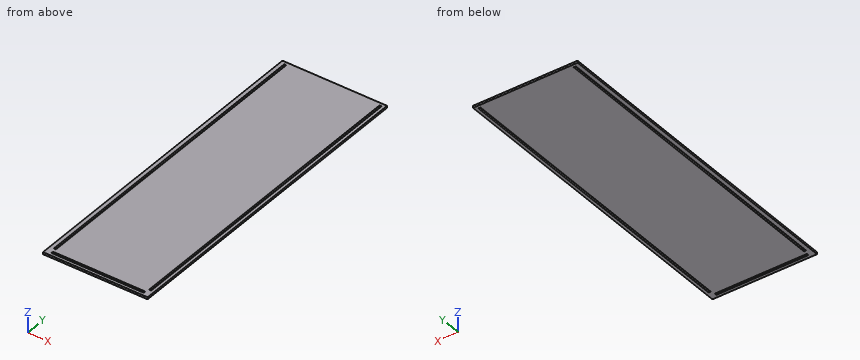
from build123d import *

# Parameters (mm, degrees)
F0_W     = 8.73125
F0_H     = 1295.4
F1_DEPTH = 8.73125


with BuildPart() as f1:
    # F0 (on Top) → F1 (new body)
    with BuildSketch(Plane.XY):
        Polygon((215.9, 673.1), (-215.9, 673.1), (-215.9, -673.1), (0, -673.1), (215.9, -673.1), (215.9, 74.258551), align=None)
        Polygon((190.5, -660.4), (0, -660.4), (-190.5, -660.4), (-190.5, -651.66875), (190.5, -651.66875), align=None, mode=Mode.SUBTRACT)
        with Locations((-194.865625, 12.70608)):
            Rectangle(F0_W, F0_H, mode=Mode.SUBTRACT)
        Polygon((203.2, 660.4), (203.2, 74.258551), (203.2, -635), (194.46875, -634.99392), (194.46875, 660.4), align=None, mode=Mode.SUBTRACT)
    extrude(amount=F1_DEPTH)


solid = f1.part
Can you work these out from the model? Positions are in its coordinate system, mm. Round coordinates to 2 decimals unless told otherwise and drop trailing zeros. Order: outer loops, then holes, each group sorted by start corner. A loop starts at its lowest first (then second) coordinate and runs counter-clockwise, first axis right, second up. Notation, with made-up numbers: (82.25, -25.5) -> (94.25, -25.5) arc R19 ccw to (94.25, -5.5) -> close; hole circle Ø4 at (16, 74.25). An arc over 180 degrees is marked (long way). Write each question's results on one line, items separated by ' | '. Start each with the question number.
Item 1: Please list where these lines run through material, in increasing order: L1, parallel to X at y = -428, z = 6; L2, parallel to Y at x = -162, z = 5.25; L3, parallel to Y at x = -192, z = 0.75.
Item 2: If we section it at A-A, the plane z = 6.75: Write out the boundary of the cut face in (x, y).
Item 3: If we section it at B-B, the plane y = -448: Write out the boundary of the cut face in (x, z).
Results:
1) L1: x = -215.9 to -199.23, -190.5 to 194.47, 203.2 to 215.9 | L2: y = -673.1 to -660.4, -651.67 to 673.1 | L3: y = -673.1 to -634.99, 660.41 to 673.1
2) outline: (-215.9, -673.1) -> (215.9, -673.1) -> (215.9, 673.1) -> (-215.9, 673.1) -> close; hole (-199.23, -634.99) -> (-190.5, -634.99) -> (-190.5, 660.41) -> (-199.23, 660.41) -> close; hole (-190.5, -660.4) -> (190.5, -660.4) -> (190.5, -651.67) -> (-190.5, -651.67) -> close; hole (194.47, -634.99) -> (203.2, -635) -> (203.2, 660.4) -> (194.47, 660.4) -> close
3) outline: (-215.9, 0) -> (-199.23, 0) -> (-199.23, 8.73) -> (-215.9, 8.73) -> close; (-190.5, 0) -> (194.47, 0) -> (194.47, 8.73) -> (-190.5, 8.73) -> close; (203.2, 0) -> (215.9, 0) -> (215.9, 8.73) -> (203.2, 8.73) -> close
